For this review, take the finished solid that the model builds, in its own axes (mm). Give positions to 0.01 mm unless a question says otherwise; leave off trailing zeros. Write each loop counter-clockwise with the first axis right and the second up, starting at its lowest first coordinate (ties: lowest second). Pieces come first, ordered by that corner, then holes. Notation, with made-up numbers: (-21, 40.25) -> (12, 40.25) arc R35 ccw to (12, 73.25) -> close; hole circle Ø1 at (-0.75, -35.75). An arc over 180 degrees is marked (long way). Write item = value, one per line.
```python
from build123d import *

# Parameters (mm, degrees)
F0_R     = 33
F1_DEPTH = 0.7
F2_R     = 5.2
F3_DEPTH = 0.7
F5_DEPTH = 0.7


with BuildPart() as f1:
    # F0 (on Top) → F1 (new body)
    with BuildSketch(Plane.XY):
        Circle(F0_R)
    extrude(amount=F1_DEPTH)

    # F2 (on face) → F3 (cut, through all)
    with BuildSketch(Plane.XY.offset(0.7)):
        Circle(F2_R)
    extrude(amount=-F3_DEPTH, mode=Mode.SUBTRACT)

    # F4 (on face) → F5 (cut, through all)
    with BuildSketch(Plane.XY.offset(0.7)):
        with BuildLine():
            Line((-1.5, 6.324555), (-1.5, 28.961181))
            ThreePointArc((-1.5, 28.961181), (-20.506097, 20.506097), (-28.961181, 1.5))
            Line((-28.961181, 1.5), (-6.324555, 1.5))
            ThreePointArc((-6.324555, 1.5), (-4.596194, 4.596194), (-1.5, 6.324555))
        make_face()
        with BuildLine():
            Line((6.324555, 1.5), (28.961181, 1.5))
            ThreePointArc((28.961181, 1.5), (20.506097, 20.506097), (1.5, 28.961181))
            Line((1.5, 28.961181), (1.5, 6.324555))
            ThreePointArc((1.5, 6.324555), (4.596194, 4.596194), (6.324555, 1.5))
        make_face()
        with BuildLine():
            ThreePointArc((1.5, -28.961181), (20.506097, -20.506097), (28.961181, -1.5))
            Line((28.961181, -1.5), (6.324555, -1.5))
            ThreePointArc((6.324555, -1.5), (4.596194, -4.596194), (1.5, -6.324555))
            Line((1.5, -6.324555), (1.5, -28.961181))
        make_face()
        with BuildLine():
            ThreePointArc((-28.961181, -1.5), (-20.506097, -20.506097), (-1.5, -28.961181))
            Line((-1.5, -28.961181), (-1.5, -6.324555))
            ThreePointArc((-1.5, -6.324555), (-4.596194, -4.596194), (-6.324555, -1.5))
            Line((-6.324555, -1.5), (-28.961181, -1.5))
        make_face()
    extrude(amount=-F5_DEPTH, mode=Mode.SUBTRACT)


solid = f1.part
```
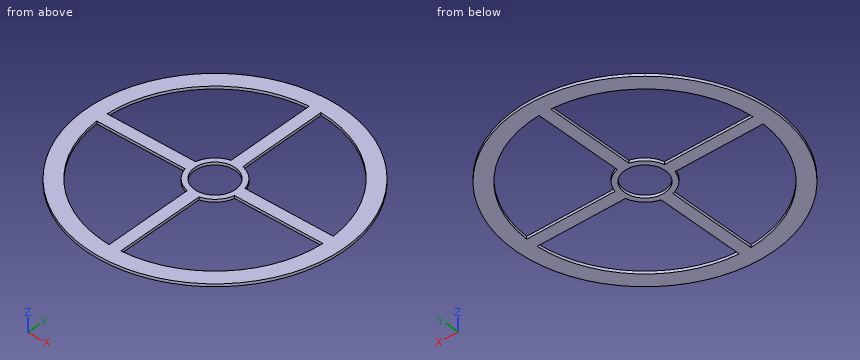
(1) Take a section at C-C (y = -21). Write out the cut boundary in (x, z), plus the area to 3 significant figures.
Answers below:
outline = (-25.46, 0) -> (-20, 0) -> (-20, 0.7) -> (-25.46, 0.7) -> close; (-1.5, 0) -> (1.5, 0) -> (1.5, 0.7) -> (-1.5, 0.7) -> close; (20, 0) -> (25.46, 0) -> (25.46, 0.7) -> (20, 0.7) -> close
area = 9.74 mm^2
(2) Take a section at A-A (z = 0.3). Write out the cut boundary in (x, y), plus the area to 3 significant figures.
Answers below:
outline = circle Ø66 at (0, 0); hole (-28.96, -1.5) arc R29 ccw to (-1.5, -28.96) -> (-1.5, -6.32) arc R6.5 cw to (-6.32, -1.5) -> close; hole (-28.96, 1.5) -> (-6.32, 1.5) arc R6.5 cw to (-1.5, 6.32) -> (-1.5, 28.96) arc R29 ccw to start; hole circle Ø10.4 at (0, 0); hole (1.5, -28.96) arc R29 ccw to (28.96, -1.5) -> (6.32, -1.5) arc R6.5 cw to (1.5, -6.32) -> close; hole (1.5, 6.32) arc R6.5 cw to (6.32, 1.5) -> (28.96, 1.5) arc R29 ccw to (1.5, 28.96) -> close
area = 1,100 mm^2
(3) Take a section at B-B (x = 0). Write out the cut boundary in (y, z).
Answers below:
outline = (-33, 0) -> (-5.2, 0) -> (-5.2, 0.7) -> (-33, 0.7) -> close; (5.2, 0) -> (33, 0) -> (33, 0.7) -> (5.2, 0.7) -> close
(4) To check wall thickness, follow probe 1 along Y at (x, z) = (-24, 0.2); probe 2 along Y at (x, z) = (-11, 0.55); probe 3 along X at (y, z) = (8, 0.1). State the ranges of each line that lie inside material, in increasing order.
Answers below:
probe_1 = -22.65 to -16.28, -1.5 to 1.5, 16.28 to 22.65
probe_2 = -31.11 to -26.83, -1.5 to 1.5, 26.83 to 31.11
probe_3 = -32.02 to -27.87, -1.5 to 1.5, 27.87 to 32.02
